Verification items for the finished model (mm, model axes). A direction names the side the tool comes from. Coordinates: 2 decimals unless noted, no trailing zeros. Write each loop counter-clockwise with the first axis right and the second up, starting at its lowest first coordinate (ties: lowest second). Pieces come first, ordered by that corner, then holes.
```python
from build123d import *

# Parameters (mm, degrees)
SKETCH1_W           = 15.4
SKETCH1_H           = 50.4
SKETCH1_W_2         = 5.4
SKETCH1_H_2         = 40.4
EXTRUDE_THIN1_DEPTH = 10
SKETCH2_W           = 15.4
SKETCH2_H           = 10
BOSS_EXTRUDE1_DEPTH = 10.8
SKETCH3_R           = 1.7
CUT_EXTRUDE1_DEPTH  = 59.022409464
FILLET1_R           = 3


with BuildPart() as part:
    # Sketch1 → Extrude-Thin1 (new body)
    with BuildSketch(Plane.XY):
        with Locations((2.7, 20.2)):
            Rectangle(SKETCH1_W, SKETCH1_H)
        with Locations((2.7, 20.2)):
            Rectangle(SKETCH1_W_2, SKETCH1_H_2, mode=Mode.SUBTRACT)
    extrude(amount=EXTRUDE_THIN1_DEPTH)

    # Sketch2 → Boss-Extrude1 (add)
    with BuildSketch(Plane(origin=(0, 45.4, 0), x_dir=(1, 0, 0), z_dir=(0, 1, 0))):
        with Locations((2.7, -5)):
            Rectangle(SKETCH2_W, SKETCH2_H)
    boss_extrude1 = extrude(amount=BOSS_EXTRUDE1_DEPTH)

    # Mirror1: Boss-Extrude1 across plane
    add(boss_extrude1.mirror(Plane.ZX.offset(20.2)))

    # Sketch3 → Cut-Extrude1 (cut, through all)
    with BuildSketch(Plane(origin=(0, 0, 0), x_dir=(-1, 0, 0), z_dir=(0, 0, -1))):
        with Locations((-2.7, 48.3)):
            Circle(SKETCH3_R)
    cut_extrude1 = extrude(amount=-CUT_EXTRUDE1_DEPTH, mode=Mode.SUBTRACT)

    # Mirror2: Cut-Extrude1 across plane
    add(cut_extrude1.mirror(Plane.ZX.offset(20.2)), mode=Mode.SUBTRACT)

    # Fillet1
    fillet1_edges = [part.edges().sort_by_distance(p)[0] for p in [
        (4.4, 48.3, 10),
        (4.4, 48.3, 0),
        (4.4, -7.9, 0),
        (4.4, -7.9, 10),
    ]]
    fillet(fillet1_edges, radius=FILLET1_R)


solid = part.part
```
1. Sectioned sample at B-B, the plane y = 38. Record the boundary of the cut face in (x, z).
2. Sectioned sample at C-C, the plane z = 5. Record the boundary of the cut face in (x, y), and give its area (3 significant figures).
3. Material ranges on L1, parallel to Y at x = 2.5, z = 4.25; L2, parallel to Y at x = 0.5, z = 8.25; L3, parallel to X at y = 11, z = 7.25, recorded low to high.
4. Gauge pin test, flat ends, axial feed: P1, Ø5.5, axis at x = 2.7, y = -7.9, coming from the +Z side; P2, Ø5.5, axis at x = 2.7, y = 48.3, coming from the -Z side. Record the tip position at first contact, or that the pin passes through.
5. Sectioned sample at A-A, the plane x = 2.7. Record the boundary of the cut face in (y, z), and give its area (3 significant figures).
6. Sectioned sample at D-D, the plane y = 48.3. Record the boundary of the cut face in (x, z), and give its area (3 significant figures).
7. Tool access check on faces 1 (the flat face through (-5, 21, 5)), 2 (the flat face through (3, 40.4, 5)). Record the directions out of +Z, -Z, +X, -X, +Y, -Y that give a thin tool (end or side, any length) a straight path to the whole face; none if there is none.
8. Draft check along Y on faces 3 (the flat face through (0, 20, 5)), 4 (the flat face through (3, 56.2, 5)), 5 (the flat face through (-1, 21, 0)), 6 (the flat face through (3, -15.8, 5)). Enter one of: pulls with the +Y half, pulls with the -Y half, needs draft (parallel to the pull), parting line crosses it, or undercut.
Outcome:
1. outline: (-5, 0) - (0, 0) - (0, 10) - (-5, 10) - close; (5.4, 0) - (10.4, 0) - (10.4, 10) - (5.4, 10) - close
2. outline: (-5, -15.8) - (10.4, -15.8) - (10.4, 56.2) - (-5, 56.2) - close; hole (0, 0) - (5.4, 0) - (5.4, 40.4) - (0, 40.4) - close; hole circle Ø3.4 at (2.7, -7.9); hole circle Ø3.4 at (2.7, 48.3)
2. area: 872 mm2
3. L1: y = -15.8 to -9.59, -6.21 to 0, 40.4 to 46.61, 49.99 to 56.2
3. L2: y = -15.8 to 0, 40.4 to 56.2
3. L3: x = -5 to 0, 5.4 to 10.4
4. P1: stops at z = 9.28
4. P2: stops at z = 0.72
5. outline: (-15.8, 0) - (-12.6, 0) arc R3 ccw to (-9.6, 3) - (-9.6, 7) arc R3 ccw to (-12.6, 10) - (-15.8, 10) - close; (-6.2, 3) arc R3 ccw to (-3.2, 0) - (0, 0) - (0, 10) - (-3.2, 10) arc R3 ccw to (-6.2, 7) - close; (40.4, 0) - (43.6, 0) arc R3 ccw to (46.6, 3) - (46.6, 7) arc R3 ccw to (43.6, 10) - (40.4, 10) - close; (50, 3) arc R3 ccw to (53, 0) - (56.2, 0) - (56.2, 10) - (53, 10) arc R3 ccw to (50, 7) - close
5. area: 233 mm2
6. outline: (-5, 0) - (-2, 0) arc R3 ccw to (1, 3) - (1, 7) arc R3 ccw to (-2, 10) - (-5, 10) - close; (4.4, 3) arc R3 ccw to (7.4, 0) - (10.4, 0) - (10.4, 10) - (7.4, 10) arc R3 ccw to (4.4, 7) - close
6. area: 112 mm2
7. face 1: +Z, -Z, -X, +Y, -Y
7. face 2: +Z, -Z
8. face 3: undercut
8. face 4: pulls with the +Y half
8. face 5: needs draft
8. face 6: pulls with the -Y half
